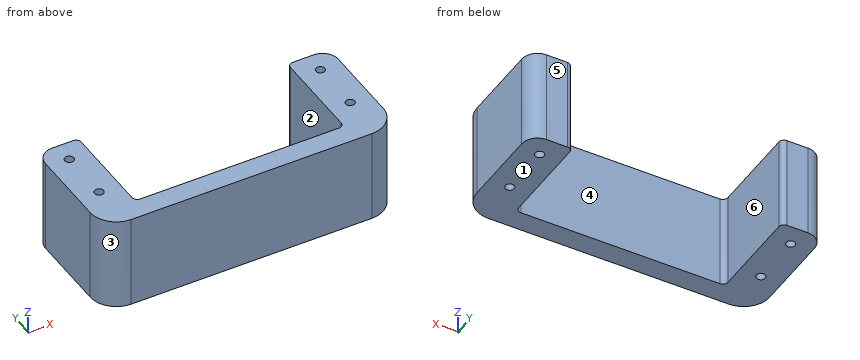
from build123d import *

# Parameters (mm, degrees)
ESQUISSE1_R        = 0.85
BOSS_EXTRU_1_DEPTH = 18
CONG_1_R           = 1
CONG_2_R           = 3
CONG_3_R           = 5


with BuildPart() as part:
    # Esquisse1 → Boss.-Extru.1 (new body)
    with BuildSketch(Plane.XY):
        Polygon((20, 23), (28, 23), (28, 0), (-28, 0), (-28, 23), (-20, 23), (-20, 4), (20, 4), align=None)
        with Locations((-24, 19)):
            Circle(ESQUISSE1_R, mode=Mode.SUBTRACT)
        with Locations((-24, 9)):
            Circle(ESQUISSE1_R, mode=Mode.SUBTRACT)
        with Locations(Location((24, 9, 0), (0, 0, 180))):
            Circle(ESQUISSE1_R, mode=Mode.SUBTRACT)
        with Locations(Location((24, 19, 0), (0, 0, 180))):
            Circle(ESQUISSE1_R, mode=Mode.SUBTRACT)
    extrude(amount=BOSS_EXTRU_1_DEPTH)

    # Congé1
    cong_1_edges = [part.edges().sort_by_distance(p)[0] for p in [
        (-20, 23, 9),
        (-20, 4, 9),
        (20, 4, 9),
        (20, 23, 9),
    ]]
    fillet(cong_1_edges, radius=CONG_1_R)

    # Congé2
    cong_2_edges = [part.edges().sort_by_distance(p)[0] for p in [
        (-28, 23, 9),
        (28, 23, 9),
    ]]
    fillet(cong_2_edges, radius=CONG_2_R)

    # Congé3
    cong_3_edges = [part.edges().sort_by_distance(p)[0] for p in [
        (28, 0, 9),
        (-28, 0, 9),
    ]]
    fillet(cong_3_edges, radius=CONG_3_R)


solid = part.part
Design review of the part built by this model. Coordinates are the model's own, in mm. Face numbers are marked on the shaded views. A direction names the side the tool comes from. Round coordinates to 2 decimals unless told otherwise and drop trailing zeros. Write each loop counter-clockwise with the first axis right and the second up, starting at its lowest first coordinate (ties: lowest second). Pieces come first, ordered by that corner, then holes. Notation, with made-up numbers: (37, -39.5) - (70, -39.5) arc R31 ccw to (70, -1.5) - close; hole circle Ø11 at (29.25, 64). An arc over 180 degrees is marked (long way). Return JSON: item names as keys, results as strings. Group by question number.
Item 1: We need section B-B on y = 9. Write out the cut boundary in (x, z), and give its area (3 significant figures).
Item 2: The part is to be moulded in two halves that separate along X. For the marked faces 3, 4, 5 and 6, say which applies: pulls with the +X half, pulls with the -X half, needs draft (parallel to the pull), parting line crosses it, or undercut.
Item 3: We need section D-D on x = 24. Write out the cut boundary in (y, z), and give its area (3 significant figures).
Item 4: We need section C-C on z = 3. Write out the cut boundary in (x, y).
Item 5: For probe 1 along Y at (x, z) = (24, 4.25); probe 2 along X at (y, z) = (8, 10.75); probe 3 along Y at (x, z) = (10, 14), list the stretches that pass through material, from the lowest coordinate up. Write a range as [from, to].
Item 6: We need section A-A on y = 13. Write out the cut boundary in (x, z), and give its area (3 significant figures).
Item 7: Machinability: for the marked faces 1 and 2, which of the approach directions +Z, -Z, +X, -X, +Y, -Y give a long, thin tool a straight path to every point of the face, cutting with its end or side? Answer none if there is none.
Item 8: Insertion check: P1, Ø2.5, axis at x = 24, y = 19, coming from the -Z side; P2, Ø9, axis at x = -3.5, z = 7.5, coming from the +Y side. Each pin has a flat end and moves straight along its axis. Give the tip position at first contact, or say it passes through.
Model answer:
{
 "1": {"outline": "(-28, 0) - (-24.85, 0) - (-24.85, 18) - (-28, 18) - close; (-23.15, 0) - (-20, 0) - (-20, 18) - (-23.15, 18) - close; (20, 0) - (23.15, 0) - (23.15, 18) - (20, 18) - close; (24.85, 0) - (28, 0) - (28, 18) - (24.85, 18) - close", "area": "227 mm²"},
 "2": {"face 3": "pulls with the -X half", "face 4": "undercut", "face 5": "needs draft", "face 6": "undercut"},
 "3": {"outline": "(0.1, 0) - (8.15, 0) - (8.15, 18) - (0.1, 18) - close; (9.85, 0) - (18.15, 0) - (18.15, 18) - (9.85, 18) - close; (19.85, 0) - (23, 0) - (23, 18) - (19.85, 18) - close", "area": "351 mm²"},
 "4": {"outline": "(-28, 5) arc R5 ccw to (-23, 0) - (23, 0) arc R5 ccw to (28, 5) - (28, 20) arc R3 ccw to (25, 23) - (21, 23) arc R1 ccw to (20, 22) - (20, 5) arc R1 cw to (19, 4) - (-19, 4) arc R1 cw to (-20, 5) - (-20, 22) arc R1 ccw to (-21, 23) - (-25, 23) arc R3 ccw to (-28, 20) - close; hole circle Ø1.7 at (-24, 9); hole circle Ø1.7 at (-24, 19); hole circle Ø1.7 at (24, 9); hole circle Ø1.7 at (24, 19)"},
 "5": {"probe 1": "y = [0.1, 8.15], [9.85, 18.15], [19.85, 23]", "probe 2": "x = [-28, -20], [20, 28]", "probe 3": "y = [0, 4]"},
 "6": {"outline": "(-28, 0) - (-20, 0) - (-20, 18) - (-28, 18) - close; (20, 0) - (28, 0) - (28, 18) - (20, 18) - close", "area": "288 mm²"},
 "7": {"face 1": "-Z, +X, -X, +Y, -Y", "face 2": "+Z, -Z, +Y"},
 "8": {"P1": "stops at z = 0", "P2": "stops at y = 4"}
}
